from build123d import *

# Parameters (mm, degrees)
SKETCH1_R           = 5
BOSS_EXTRUDE1_DEPTH = 30
SKETCH2_R           = 6.5
BOSS_EXTRUDE2_DEPTH = 2
SKETCH3_R           = 6.5
BOSS_EXTRUDE3_DEPTH = 8


with BuildPart() as part:
    # Sketch1 → Boss-Extrude1 (new body)
    with BuildSketch(Plane(origin=(0, 0, 0), x_dir=(1, 0, 0), z_dir=(0, 1, 0))):
        Circle(SKETCH1_R)
    extrude(amount=BOSS_EXTRUDE1_DEPTH)

    # Sketch2 → Boss-Extrude2 (add)
    with BuildSketch(Plane(origin=(0, 30, 0), x_dir=(1, 0, 0), z_dir=(0, 1, 0))):
        Circle(SKETCH2_R)
    extrude(amount=BOSS_EXTRUDE2_DEPTH)

    # Sketch3 → Boss-Extrude3 (add)
    with BuildSketch(Plane(origin=(0, 32, 0), x_dir=(1, 0, 0), z_dir=(0, 1, 0))):
        Circle(SKETCH3_R)
        Polygon((5.196152423, 0), (2.598076211, 4.5), (-2.598076211, 4.5), (-5.196152423, 0), (-2.598076211, -4.5), (2.598076211, -4.5), align=None, mode=Mode.SUBTRACT)
    extrude(amount=BOSS_EXTRUDE3_DEPTH)


solid = part.part
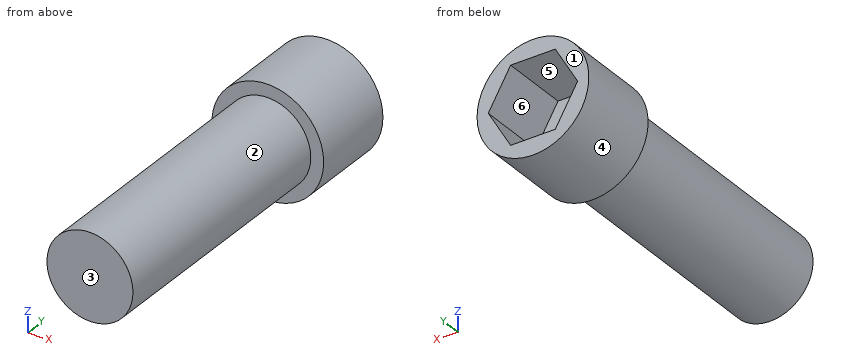
Source: CAD feature listing. Evaluate the final solid. Frame: model axes, mm. Face numbers are marked on the shaded views. A direction names the side the tool comes from. Round coordinates to 2 decimals unless told otherwise and drop trailing zeros. Loops run counter-clockwise (first coordinate to the right, second up) from the corner with the lowest first, then second, coordinate; pieces in that order, holes last. Notation, with made-up numbers: M 12.5,11.5 L 57.5,11.5 A22 ccw 57.5,45.5 Z; hole C -40,89.5 d9. An arc over 180 degrees is marked long. Answer as CSV lines item,"result".
Q1. Cut plane A-A (x = 0). Return the cut outline in (y, z), plus the area to 3 significant figures.
Verdict:
outline,"M 0,-5 L 30,-5 L 30,-6.5 L 40,-6.5 L 40,-4.5 L 32,-4.5 L 32,4.5 L 40,4.5 L 40,6.5 L 30,6.5 L 30,5 L 0,5 Z"
area,"358 mm^2"
Q2. Cut plane B-B (z = -3.5). Return the cut outline in (x, y).
Verdict:
outline,"M -5.48,30 L -3.57,30 L -3.57,0 L 3.57,0 L 3.57,30 L 5.48,30 L 5.48,40 L 3.18,40 L 3.18,32 L -3.18,32 L -3.18,40 L -5.48,40 Z"
Q3. Contact query for flat-ended pins moving along their axis: pin 1 (3 mm diameter, centred on x = 2, z = -4, fed in from +Y); pin 2 (6 mm diameter, centred on x = 1, z = -0.5, fed in from +Y); pin 3 (6 mm diameter, centred on y = 10, z = -3.5, fed in from +X); pin 4 (2 mm diameter, centred on y = 13, z = -4, fed in from +X). Output: stop coordinate, or through.
Verdict:
pin 1,"stops at y = 40"
pin 2,"stops at y = 32"
pin 3,"stops at x = 4.97"
pin 4,"stops at x = 4"
Q4. Pull-direction query (Z, two-part tool) for the marked faces 3, 4, 5 and 6; classes: +Z half, -Z half, draft (parallel to the pull), parting line (faces both ways), or undercut.
Verdict:
face 3,"draft"
face 4,"parting line"
face 5,"undercut"
face 6,"undercut"
Q5. Reachability of the marked faces 1 and 2 from +Z, -Z, +X, -X, +Y, -Y: full face, straight path, thin tool, end or side. Return the list, or none.
Verdict:
face 1,"+Z, -Z, +X, -X, +Y"
face 2,"-Y"
Q6. Line query: line 1 along Y through (x, z) = (2.75, -4.75); line 2 along Y through (x, z) = (-2, -0.75); line 3 along Z through (x, y) = (-3.25, 36.5). Output: solid intervals per line, ascending.
Verdict:
line 1,"y = 30 to 40"
line 2,"y = 0 to 32"
line 3,"z = -5.63 to -3.37, 3.37 to 5.63"
Q7. Cut plane C-C (y = 7). Return the cut outline in (x, z).
Verdict:
outline,"C 0,0 d10"
